The listing builds one solid part. Answer for the finished solid, in the listing's coordinates (mm). A direction names the side the tool comes from. Round coordinates to 2 decimals unless told otherwise and drop trailing zeros. Order: outer loops, then holes, each group sorted by start corner. A loop starts at its lowest first (then second) coordinate and runs counter-clockwise, first axis right, second up. Notation, with made-up numbers: (21.25, 27) - (47.25, 27) arc R16 ccw to (47.25, 37) - close; hole circle Ø5 at (-28, -21). An arc over 180 degrees is marked (long way). Use CSV: the item, a comma, the result in double quotes. Start each with the question number.
Item 1: Determine the mould class of faces 1 (the cylindrical face through (-1.172, -8.923, -2.007)), 2 (the flat face through (-7, -6, 2.5)), 3 (the cylindrical face through (-11.99, 0.53, 0.32)) for opening direction X: +X half, -X half, draft (parallel to the pull), parting line (faces both ways), or undercut.
Item 2: For faces 4 (the cylindrical face through (4.57, -7.167, -2.007)), 5 (the cylindrical face through (-7.493, 0.33, -0.035)), 6 (the cylindrical face through (4.57, 7.167, 2.007)), determine the directions among +Z, -Z, +X, -X, +Y, -Y from which every point of the face is accessible in a straight line to the end or side of a thin tool.
Item 3: Flat-ended cylindrical pins translate along their axes: P1, Ø1, axis at y = 7.5, z = -1, coming from the -X side; P2, Ø1.5, axis at y = -2.5, z = -1, coming from the -X side. Find the tip coordinate at first contact, or state that the pin passes through.
Item 4: Straight lines are drawn through the part: line 1 along Y through (x, z) = (0, -1.75); line 2 along Y through (x, z) = (0, 2); line 3 along Y through (x, z) = (0, -0.65). For each, find the intervals that lie inside material, in ascending order. Write a range as [from, to].
Item 5: Find section C-C, the plane z = 0.95. Give the vertices of the cut face in (x, y).
```python
from build123d import *

# Parameters (mm, degrees)
F0_R     = 12
F0_R_2   = 7.5
F1_DEPTH = 2.5
F2_R     = 0.5
F3_R     = 13
F3_R_2   = 10
F4_DEPTH = 1.1
F5_R     = 9
F5_R_2   = 8.5
F6_DEPTH = 1
F7_R     = 9
F7_R_2   = 8.5
F8_DEPTH = 1


with BuildPart() as f1:
    # F0 (on Top) → F1 (new body, symmetric)
    with BuildSketch(Plane.XY):
        Circle(F0_R)
        Circle(F0_R_2, mode=Mode.SUBTRACT)
    extrude(amount=F1_DEPTH, both=True)

    # F2
    f2_edges = [f1.edges().sort_by_distance(p)[0] for p in [
        (-12, 0, 2.5),
    ]]
    fillet(f2_edges, radius=F2_R)

    # F3 (on face) → F4 (join)
    with BuildSketch(Plane(origin=(0, 0, -2.5), x_dir=(1, 0, 0), z_dir=(0, 0, -1))):
        Circle(F3_R)
        Circle(F3_R_2, mode=Mode.SUBTRACT)
    extrude(amount=-F4_DEPTH)

    # F5 (on face) → F6 (cut)
    with BuildSketch(Plane(origin=(0, 0, -2.5), x_dir=(1, 0, 0), z_dir=(0, 0, -1))):
        Circle(F5_R)
        Circle(F5_R_2, mode=Mode.SUBTRACT)
    extrude(amount=-F6_DEPTH, mode=Mode.SUBTRACT)

    # F7 (on face) → F8 (cut)
    with BuildSketch(Plane.XY.offset(2.5)):
        Circle(F7_R)
        Circle(F7_R_2, mode=Mode.SUBTRACT)
    extrude(amount=-F8_DEPTH, mode=Mode.SUBTRACT)


solid = f1.part
```
Worked out:
1,face 1,"undercut"
1,face 2,"draft"
1,face 3,"parting line"
2,face 4,"-Z"
2,face 5,"+Z, -Z"
2,face 6,"+Z"
3,P1,"stops at x = -10.82"
3,P2,"stops at x = -12.87"
4,line 1,"y = [-13, -9], [-8.5, -7.5], [7.5, 8.5], [9, 13]"
4,line 2,"y = [-12, -9], [-8.5, -7.5], [7.5, 8.5], [9, 12]"
4,line 3,"y = [-12, -7.5], [7.5, 12]"
5,outline,"circle Ø24 at (0, 0); hole circle Ø15 at (0, 0)"
